```python
from build123d import *

# Parameters (mm, degrees)
ESBO_O1_R                = 5
ESBO_O1_R_2              = 2.5
RESSALTO_EXTRUS_O1_DEPTH = 10


with BuildPart() as part:
    # Esboço1 → Ressalto-extrusão1 (new body)
    with BuildSketch(Plane.XY):
        with BuildLine():
            Line((-6, -76), (-6, -13.747727085))
            ThreePointArc((-6, -13.747727085), (-5.740251485, 13.858192988), (13.963751735, -5.47847036))
            Line((13.963751735, -5.47847036), (74.52152964, -66.036248265))
            ThreePointArc((74.52152964, -66.036248265), (93.858192988, -85.740251485), (66.252272915, -86))
            Line((66.252272915, -86), (4, -86))
            ThreePointArc((4, -86), (-3.071067812, -83.071067812), (-6, -76))
        make_face()
        Circle(ESBO_O1_R, mode=Mode.SUBTRACT)
        with Locations((0, -30)):
            Circle(ESBO_O1_R_2, mode=Mode.SUBTRACT)
        with Locations((0, -56)):
            Circle(ESBO_O1_R_2, mode=Mode.SUBTRACT)
        with Locations((4, -76)):
            Circle(ESBO_O1_R_2, mode=Mode.SUBTRACT)
        with Locations((24, -80)):
            Circle(ESBO_O1_R_2, mode=Mode.SUBTRACT)
        with Locations((50, -80)):
            Circle(ESBO_O1_R_2, mode=Mode.SUBTRACT)
        with Locations((80, -80)):
            Circle(ESBO_O1_R, mode=Mode.SUBTRACT)
        with Locations((28.284271247, -28.284271247)):
            Circle(ESBO_O1_R_2, mode=Mode.SUBTRACT)
        with Locations((51.715728753, -51.715728753)):
            Circle(ESBO_O1_R_2, mode=Mode.SUBTRACT)
        with BuildLine():
            Line((21.291616466, -74), (59.009632228, -74))
            ThreePointArc((59.009632228, -74), (61.781270826, -72.148050297), (61.130952572, -68.878679656))
            Line((61.130952572, -68.878679656), (11.121320344, -18.869047428))
            ThreePointArc((11.121320344, -18.869047428), (7.851949703, -18.218729174), (6, -20.990367772))
            Line((6, -20.990367772), (6, -58.708383534))
            ThreePointArc((6, -58.708383534), (6.602084238, -60.511159172), (8.166666667, -61.590319612))
            ThreePointArc((8.166666667, -61.590319612), (14.606601718, -65.393398282), (18.409680388, -71.833333333))
            ThreePointArc((18.409680388, -71.833333333), (19.488840828, -73.397915762), (21.291616466, -74))
        make_face(mode=Mode.SUBTRACT)
    extrude(amount=RESSALTO_EXTRUS_O1_DEPTH)


solid = part.part
```
Here's how the part is built. I have some questions about the finished solid (model axes, mm). A direction names the side the tool comes from. Coordinates: 2 decimals unless noted, no trailing zeros. Order: outer loops, then holes, each group sorted by start corner. A loop starts at its lowest first (then second) coordinate and runs counter-clockwise, first axis right, second up.
1) We'd pull the mould along Y, two halves only. Please class faces 1 (the face through (36, -40, 10)), 2 (the face through (21.5, -79.9, 4.9)), 3 (the face through (36, -86, 5)): +Y half, -Y half, draft (parallel to the pull), parting line (faces both ways), or undercut.
2) Imagine slicing it at A-A on x = 80. List the corners of the cut face in (y, z) for me.
3) Will these pins go through, and if not, where does the flat tip stop? pin 1 (4.5 mm diameter, centred on x = 0, y = -30, fed in from +Z); pin 2 (4 mm diameter, centred on x = 18.5, z = 6, fed in from -Y); pin 3 (6 mm diameter, centred on x = 28.28, y = -28.28, fed in from +Z); pin 4 (2 mm diameter, centred on x = 23.5, z = 8.5, fed in from +Y).
4) Which directions (+Z, -Z, +X, -X, +Y, -Y) give clear straight access to the entire face, cutting with the end or side of a thin tool? Please do faces 4 (the face through (-6, -45, 5)), 5 (the face through (36, -40, 0)), 6 (the face through (7.9, -18.2, 4.9)).
5) Imagine slicing it at D-D on x = 0. List the corners of the cut face in (y, z) for me.
6) Imagine slicing it at B-B on y = -56. List the corners of the cut face in (x, z) for me, and give its area (3 significant figures).
7) Imagine slicing it at C-C on y = -80. List the corners of the cut face in (x, z) for me.
8) I need wall thicknesses on line 1 (Y direction, x = 80, z = 3.75); line 2 (Y direction, x = 0, z = 5.5); line 3 (Y direction, x = -2, z = 4). Which ranges of each line are inside material? Lowest first, please.
Response values:
1. face 1: draft
1. face 2: undercut
1. face 3: -Y half
2. outline: (-95, 0) - (-85, 0) - (-85, 10) - (-95, 10) - close; (-75, 0) - (-65, 0) - (-65, 10) - (-75, 10) - close
3. pin 1: passes through
3. pin 2: stops at y = -86
3. pin 3: stops at z = 10
3. pin 4: stops at y = -14.01
4. face 4: +Z, -Z, -X, -Y
4. face 5: -Z, +X, -X, +Y, -Y
4. face 6: +Z, -Z
5. outline: (-85.17, 0) - (-58.5, 0) - (-58.5, 10) - (-85.17, 10) - close; (-53.5, 0) - (-32.5, 0) - (-32.5, 10) - (-53.5, 10) - close; (-27.5, 0) - (-5, 0) - (-5, 10) - (-27.5, 10) - close; (5, 0) - (15, 0) - (15, 10) - (5, 10) - close
6. outline: (-6, 0) - (-2.5, 0) - (-2.5, 10) - (-6, 10) - close; (2.5, 0) - (6, 0) - (6, 10) - (2.5, 10) - close; (48.25, 0) - (64.49, 0) - (64.49, 10) - (48.25, 10) - close
6. area: 232 mm2
7. outline: (-5.17, 0) - (21.5, 0) - (21.5, 10) - (-5.17, 10) - close; (26.5, 0) - (47.5, 0) - (47.5, 10) - (26.5, 10) - close; (52.5, 0) - (75, 0) - (75, 10) - (52.5, 10) - close; (85, 0) - (95, 0) - (95, 10) - (85, 10) - close
8. line 1: y = -95 to -85, -75 to -65
8. line 2: y = -85.17 to -58.5, -53.5 to -32.5, -27.5 to -5, 5 to 15
8. line 3: y = -84 to -57.5, -54.5 to -31.5, -28.5 to -4.58, 4.58 to 14.87
